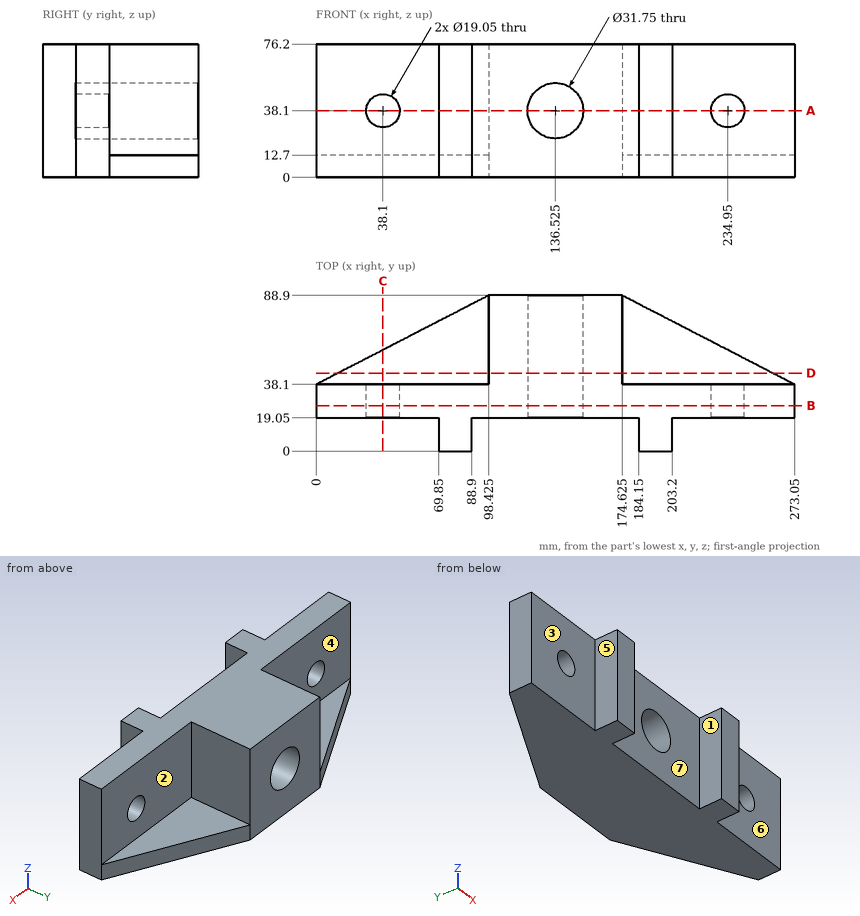
Can you work these out from the drawing? Everything is in mm from the part's minimum corner. A direction names the side the tool comes from. Round coordinates to 2 decimals unless told otherwise and drop trailing zeros. Order: outer loops, then holes, each group sorted by start corner. A loop starts at its lowest first (then second) coordinate and runs counter-clockwise, first axis right, second up. Notation, with made-up numbers: M 21.5,-19 L 47.5,-19 A8 ccw 47.5,-15 Z; hole C 78.5,44 d1. An arc over 180 degrees is marked long. Answer as CSV lines item,"result".
Item 1: Please list where these lines run through material, in increasing order: L1, parallel to X at y = 26, z = 38; L2, parallel to X at y = 79, z = 39 (3 decimals); L3, parallel to X at y = 10.5, z = 21.5. Write a range as [from, to].
From the geometry:
L1,"[0, 28.58], [47.62, 120.65], [152.4, 225.43], [244.47, 273.05]"
L2,"[98.425, 120.676], [152.374, 174.625]"
L3,"[69.85, 88.9], [184.15, 203.2]"
Item 2: Imagine slicing it at C-C on x = 38.1. List the corners of the cut face in (y, z) for me (3 decimals).
From the geometry:
outline,"M 19.05,0 L 57.765,0 L 57.765,12.7 L 38.1,12.7 L 38.1,28.575 L 19.05,28.575 Z; M 19.05,47.625 L 38.1,47.625 L 38.1,76.2 L 19.05,76.2 Z"
Item 3: For pin 1 (9.5 mm diameter, centred on y = 6.5, z = 50, fed in from +X); pin 2 (1 mm diameter, centred on y = 76.5, z = 15.5, fed in from -X) (3 decimals); pin 3 (19 mm diameter, centred on x = 34, z = 40.5, fed in from +Y); pin 4 (15 mm diameter, centred on x = 38.1, z = 38.1, fed in from -Y), each with a flat end and sliding along its axis, tell me the tip position at first contact or that it passes through.
From the geometry:
pin 1,"x = 203.2"
pin 2,"x = 98.425"
pin 3,"y = 38.1"
pin 4,"through"
Item 4: Imagine slicing it at A-A on z = 38.1. List the corners of the cut face in (x, y) for me (3 decimals), and give its area (3 significant figures).
From the geometry:
outline,"M 0,19.05 L 28.575,19.05 L 28.575,38.1 L 0,38.1 Z; M 47.625,19.05 L 69.85,19.05 L 69.85,0 L 88.9,0 L 88.9,19.05 L 120.65,19.05 L 120.65,88.9 L 98.425,88.9 L 98.425,38.1 L 47.625,38.1 Z; M 152.4,19.05 L 184.15,19.05 L 184.15,0 L 203.2,0 L 203.2,19.05 L 225.425,19.05 L 225.425,38.1 L 174.625,38.1 L 174.625,88.9 L 152.4,88.9 Z; M 244.475,19.05 L 273.05,19.05 L 273.05,38.1 L 244.475,38.1 Z"
area,"6,850 mm2"
Item 5: Imagine slicing it at B-B on y = 26. List the corners of the cut face in (x, z) for me (3 decimals), and give its area (3 significant figures).
From the geometry:
outline,"M 0,0 L 273.05,0 L 273.05,76.2 L 0,76.2 Z; hole C 38.1,38.1 d19.05; hole C 136.525,38.1 d31.75; hole C 234.95,38.1 d19.05"
area,"19,400 mm2"
Item 6: We'd pull the mould along X, two halves only. Please class the marked faces 5, 6 and 7: +X half, -X half, draft (parallel to the pull), parting line (faces both ways), or undercut.
From the geometry:
face 5,"-X half"
face 6,"draft"
face 7,"undercut"
Item 7: Which directions (+Z, -Z, +X, -X, +Y, -Y) give clear straight access to the entire face, cutting with the end or side of a thin tool? Please do the marked faces 1, 2, 3 and 4.
From the geometry:
face 1,"+Z, -Z, -Y"
face 2,"+Z, +X, +Y"
face 3,"+Z, -Z, -X, -Y"
face 4,"+Z, -X, +Y"
Item 8: Imagine slicing it at D-D on y = 44.5. List the corners of the cut face in (x, z) for me (3 decimals).
From the geometry:
outline,"M 12.4,0 L 260.65,0 L 260.65,12.7 L 174.625,12.7 L 174.625,76.2 L 98.425,76.2 L 98.425,12.7 L 12.4,12.7 Z; hole C 136.525,38.1 d31.75"
